Check sheet for the modelled part. Datum: model origin and axes. Units: mm. A direction names the side the tool comes from. Give positions to 0.01 mm unless a question says otherwise; leave off trailing zeros. Loops run counter-clockwise (first coordinate to the right, second up) from the corner with the lowest first, then second, coordinate; pieces in that order, holes last. Notation, with made-up numbers: (78, 46) - (97, 46) arc R12 ccw to (97, 54) - close; hole circle Ø4 at (18, 12). An arc over 180 degrees is marked (long way). Use CSV: the item, a comma, the result in double quotes.
from build123d import *

# Parameters (mm, degrees)
SKETCH1_R           = 13.7541
BOSS_EXTRUDE1_DEPTH = 11.7856
SKETCH2_R           = 14.9225
BOSS_EXTRUDE2_DEPTH = 21.1582
SKETCH3_R           = 11.6205
BOSS_EXTRUDE3_DEPTH = 8.5598
SKETCH4_R           = 21.082
BOSS_EXTRUDE4_DEPTH = 4.2164
SKETCH6_R           = 19.2024
SKETCH5_R           = 23.4315
SKETCH8_R           = 10.2235
SKETCH9_R           = 10.2235
BOSS_EXTRUDE5_DEPTH = 5.461
SKETCH11_R          = 4.9911
BOSS_EXTRUDE6_DEPTH = 17.78
FILLET1_R           = 5.08


with BuildPart() as part:
    # Sketch1 → Boss-Extrude1 (new body)
    with BuildSketch(Plane(origin=(0, 0, 0), x_dir=(1, 0, 0), z_dir=(0, 1, 0))):
        with Locations(Location((0, 0, 0), (0, 0, 270))):
            Circle(SKETCH1_R)
    extrude(amount=BOSS_EXTRUDE1_DEPTH)

    # Sketch2 → Boss-Extrude2 (add)
    with BuildSketch(Plane(origin=(0, 11.7856, 0), x_dir=(1, 0, 0), z_dir=(0, 1, 0))):
        with Locations(Location((0, 0, 0), (0, 0, 270))):
            Circle(SKETCH2_R)
    extrude(amount=BOSS_EXTRUDE2_DEPTH)

    # Sketch3 → Boss-Extrude3 (add)
    with BuildSketch(Plane(origin=(0, 32.9438, 0), x_dir=(1, 0, 0), z_dir=(0, 1, 0))):
        with Locations(Location((0, 0, 0), (0, 0, 270))):
            Circle(SKETCH3_R)
    extrude(amount=BOSS_EXTRUDE3_DEPTH)

    # Sketch4 → Boss-Extrude4 (add)
    with BuildSketch(Plane(origin=(0, 41.5036, 0), x_dir=(1, 0, 0), z_dir=(0, 1, 0))):
        with Locations(Location((0, 0, 0), (0, 0, 270))):
            Circle(SKETCH4_R)
    extrude(amount=BOSS_EXTRUDE4_DEPTH)

    # Sketch6 → Loft1 section 0
    with BuildSketch(Plane(origin=(0, 75.9206, 0), x_dir=(1, 0, 0), z_dir=(0, 1, 0))):
        Circle(SKETCH6_R)
    # Sketch5 → Loft1 section 1
    with BuildSketch(Plane(origin=(0, 45.72, 0), x_dir=(1, 0, 0), z_dir=(0, 1, 0))):
        Circle(SKETCH5_R)
    loft()

    # Sketch8 → section 1 of loft2
    with BuildSketch(Plane(origin=(0, 83.9216, 0), x_dir=(1, 0, 0), z_dir=(0, 1, 0)), mode=Mode.PRIVATE) as loft2_s1:
        Circle(SKETCH8_R)
    # loft up to a face of the part (loft2)
    loft([Face(Wire([part.edges().sort_by_distance((-13.144947347, 75.9206, -13.997947171))[0]])), loft2_s1.sketch])

    # Sketch9 → Boss-Extrude5 (add)
    with BuildSketch(Plane(origin=(0, 83.9216, 0), x_dir=(1, 0, 0), z_dir=(0, 1, 0))):
        with Locations(Location((0, 0, 0), (0, 0, 270))):
            Circle(SKETCH9_R)
    extrude(amount=BOSS_EXTRUDE5_DEPTH)

    # Sketch11 → Boss-Extrude6 (add)
    with BuildSketch(Plane(origin=(0, 89.3826, 0), x_dir=(1, 0, 0), z_dir=(0, 1, 0))):
        with Locations(Location((0, 0, 0), (0, 0, 270))):
            Circle(SKETCH11_R)
    extrude(amount=BOSS_EXTRUDE6_DEPTH)

    # Fillet1
    fillet1_edges = [part.edges().sort_by_distance(p)[0] for p in [
        (-7.229106177, 83.9216, -7.229106177),
    ]]
    fillet(fillet1_edges, radius=FILLET1_R)


solid = part.part
1. Scan lines: line 1 along Y through (x, z) = (-3, -5); line 2 along Y through (x, z) = (-4, 13); line 3 along Y through (x, z) = (11, -10). Record each from-to range of solid material in increasing order.
Completed:
line 1,"y = 0 to 89.38"
line 2,"y = 0 to 32.94, 41.5 to 80.91"
line 3,"y = 11.79 to 32.94, 41.5 to 79.78"
2. Release check for a two-part mould opening along Y. For faces 1 (the face through (-9, 32.944, 8)), 2 (the face through (-9, 41.504, 9)), 3 (the face through (-13.239, 22.217, 6.886)), 4 (the face through (5, 89.383, 2)) record: released by +Y, released by -Y, zero draft, split by the parting line, or undercut.
Completed:
face 1,"undercut"
face 2,"undercut"
face 3,"zero draft"
face 4,"released by +Y"
3. Sectioned sample at B-B, the plane y = 16.5. Record the boundary of the cut face in (x, z) (1 decimal).
Completed:
outline,"circle Ø29.8 at (0, 0)"
4. Go/stop test with flat-tipped pins: pin 1 Ø5 at (x, y) = (13, 11.5) entering from -Z; pin 2 Ø8 at (x, y) = (-13.5, 56) entering from -Z; pin 3 Ø1.5 at (y, z) = (52, -10.5) entering from +X. Record where each tip stops, or that it passes through.
Completed:
pin 1,"stops at z = -10.59"
pin 2,"stops at z = -19.93"
pin 3,"stops at x = 20.35"
5. Sectioned sample at A-A, the plane y = 91. Record the boundary of the cut face in (x, z).
Completed:
outline,"circle Ø9.98 at (0, 0)"
6. Set-up check for faces 5 (the face through (-4.4, 11.786, 13.2)), 6 (the face through (-11.344, 37.164, -2.519)), 7 (the face through (-4.872, 98.148, -1.082)): record each of +Z, -Z, +X, -X, +Y, -Y from which the full face is reachable in a straight line by a thin tool's end or side.
Completed:
face 5,"-Y"
face 6,"none"
face 7,"+Y"
